Read the model definition and answer for the solid it produces. Units are mm, in the model's axes. Face numbers are marked on the shaded views. A direction names the side the tool comes from. Coordinates: 2 decimals unless noted, no trailing zeros. Loops run counter-clockwise (first coordinate to the right, second up) from the corner with the lowest first, then second, coordinate; pieces in that order, holes last. Notation, with made-up numbers: (37.25, -30.75) - (77.25, -30.75) arc R21 cw to (77.25, -9.75) - close; hole circle Ø3 at (-2, -9.5). An arc over 180 degrees is marked (long way). Use one line per item in the form item = value.
from build123d import *

# Parameters (mm, degrees)
EXTRUDE_2_DEPTH                = 5
SKETCH_4_W                     = 8.676470589
SKETCH_4_H                     = 35
SKETCH_4_W_2                   = 8.676470588
EXTRUDE_15_DEPTH               = 35
CUT_EXTRUDE_1_DEPTH            = 45
SKETCH_6_R                     = 15
CUT_EXTRUDE_2_DEPTH            = 45
FILLET_1_R                     = 5
EXTRUDE_START                  = -1
SKETCH_7_R                     = 15
SKETCH_7_R_2                   = 13
EXTRUDE_16_DEPTH               = 1
SPLIT_BODIES_1_SURFACE_1_BACK  = 86
SPLIT_BODIES_1_SURFACE_1_DEPTH = 172
SPLIT_BODIES_1_SURFACE_2_BACK  = 86
SPLIT_BODIES_1_SURFACE_2_DEPTH = 172
SKETCH_17_W                    = 3
SKETCH_17_H                    = 13
EXTRUDE_20_DEPTH               = 42
HOLE_WIZARD_1_D                = 4.3
HOLE_WIZARD_1_DEPTH            = 5
HOLE_WIZARD_1_CBORE_D          = 10
HOLE_WIZARD_1_CBORE_DEPTH      = 0.5
HOLE_WIZARD_1_TIP              = 1.291850331
EXTRUDE_21_DEPTH               = 3
SKETCH_33_R                    = 1.6
CUT_EXTRUDE_3_DEPTH            = 3
EXTRUDE_22_DEPTH               = 5
FILLET_2_R                     = 6


with BuildPart() as part:
    # 草图2 → 凸台-拉伸2 (new body)
    with BuildSketch(Plane.XY):
        Polygon((7.726423565, 24.338235294), (-14.773576435, 24.338235294), (-14.773576435, -35.661764706), (7.726423565, -35.661764706), (7.726423565, -23.161764706), (-6.097105846, -23.161764706), (-6.097105846, 11.838235294), (7.726423565, 11.838235294), align=None)
        Polygon((30.226423565, 24.338235294), (7.726423565, 24.338235294), (7.726423565, 11.838235294), (21.549952977, 11.838235294), (21.549952977, -23.161764706), (7.726423565, -23.161764706), (7.726423565, -35.661764706), (30.226423565, -35.661764706), align=None)
    extrude(amount=EXTRUDE_2_DEPTH)

    # 草图4 → 凸台-拉伸15 (add)
    with BuildSketch(Plane.XY.offset(5)):
        with Locations((-10.435341141, -5.661764706)):
            Rectangle(SKETCH_4_W, SKETCH_4_H)
        with Locations((25.888188271, -5.661764706)):
            Rectangle(SKETCH_4_W_2, SKETCH_4_H)
    extrude(amount=EXTRUDE_15_DEPTH)

    # 草图5 → 切除-拉伸1 (cut)
    with BuildSketch(Plane.ZY.offset(14.773576435)):
        with BuildLine():
            Line((40, -23.161764706), (40, -5.661764706))
            ThreePointArc((40, -5.661764706), (34.874368671, -18.036133377), (22.5, -23.161764706))
            Line((22.5, -23.161764706), (40, -23.161764706))
        make_face()
        with BuildLine():
            ThreePointArc((22.5, 11.838235294), (34.874368671, 6.712603965), (40, -5.661764706))
            Line((40, -5.661764706), (40, 11.838235294))
            Line((40, 11.838235294), (22.5, 11.838235294))
        make_face()
    extrude(amount=-CUT_EXTRUDE_1_DEPTH, mode=Mode.SUBTRACT)

    # 草图6 → 切除-拉伸2 (cut)
    with BuildSketch(Plane.ZY.offset(14.773576435)):
        with Locations((22.5, -5.661764706)):
            Circle(SKETCH_6_R)
    extrude(amount=-CUT_EXTRUDE_2_DEPTH, mode=Mode.SUBTRACT)

    # 圆角1
    fillet_1_edges = [part.edges().sort_by_distance(p)[0] for p in [
        (-6.097105846, 11.838235294, 2.5),
        (-6.097105846, -23.161764706, 2.5),
        (21.549952977, -23.161764706, 2.5),
        (21.549952977, 11.838235294, 2.5),
    ]]
    fillet(fillet_1_edges, radius=FILLET_1_R)

    # 草图7 → 凸台-拉伸16 (add)
    with BuildSketch(Plane(origin=(-6.097105846, 0, 0), x_dir=(0, 0, -1), z_dir=(1, 0, 0)).offset(EXTRUDE_START)):
        with Locations(Location((-22.5, -5.661764706, 0), (0, 0, 180))):
            Circle(SKETCH_7_R)
        with Locations((-22.5, -5.661764706)):
            Circle(SKETCH_7_R_2, mode=Mode.SUBTRACT)
    extrude(amount=EXTRUDE_16_DEPTH)


with BuildPart() as body_2:
    # Split Bodies 1: the piece behind the surface
    add(part.part)
    # Split Bodies 1 surface: a surface, the sketch's curves swept straight by 172 mm
    with BuildLine(Plane.XY.offset(5).offset(-SPLIT_BODIES_1_SURFACE_1_BACK), mode=Mode.PRIVATE) as split_bodies_1_surface_1_path:
        Line((7.726423565, 24.338235294), (7.726423565, -35.661764706))
    split_bodies_1_surface_1 = Shell.extrude(split_bodies_1_surface_1_path.wire(), (0 * SPLIT_BODIES_1_SURFACE_1_DEPTH, 0 * SPLIT_BODIES_1_SURFACE_1_DEPTH, 1 * SPLIT_BODIES_1_SURFACE_1_DEPTH))
    split(bisect_by=split_bodies_1_surface_1, keep=Keep.BOTTOM)


with BuildPart() as part_1:
    add(part.part)

    # Split Bodies 1: split by a surface, the side it looks to stays
    # Split Bodies 1 surface: a surface, the sketch's curves swept straight by 172 mm
    with BuildLine(Plane.XY.offset(5).offset(-SPLIT_BODIES_1_SURFACE_2_BACK), mode=Mode.PRIVATE) as split_bodies_1_surface_2_path:
        Line((7.726423565, 24.338235294), (7.726423565, -35.661764706))
    split_bodies_1_surface_2 = Shell.extrude(split_bodies_1_surface_2_path.wire(), (0 * SPLIT_BODIES_1_SURFACE_2_DEPTH, 0 * SPLIT_BODIES_1_SURFACE_2_DEPTH, 1 * SPLIT_BODIES_1_SURFACE_2_DEPTH))
    split(bisect_by=split_bodies_1_surface_2, keep=Keep.TOP)

    # 草图17 → 凸台-拉伸20 (add)
    with BuildSketch(Plane.XY.offset(5)):
        with Locations((28.726423565, -34.661764706)):
            Rectangle(SKETCH_17_W, SKETCH_17_H)
        with Locations((28.726423565, 25.338235294)):
            Rectangle(SKETCH_17_W, SKETCH_17_H)
    extrude(amount=EXTRUDE_20_DEPTH)

    # 打孔尺寸(%根据六角头螺)栓 全螺纹的类型1
    with Locations(Plane(origin=(18.226423565, 18.088235294, 5), x_dir=(1, 0, 0), z_dir=(0, 0, 1))):
        with Locations((0, 0), (0, -47.5)):
            CounterBoreHole(HOLE_WIZARD_1_D / 2, HOLE_WIZARD_1_CBORE_D / 2, HOLE_WIZARD_1_CBORE_DEPTH, depth=HOLE_WIZARD_1_DEPTH)
            with Locations((0, 0, -(HOLE_WIZARD_1_DEPTH + HOLE_WIZARD_1_TIP / 2))):  # 118° drill point
                Cone(0, HOLE_WIZARD_1_D / 2, HOLE_WIZARD_1_TIP, mode=Mode.SUBTRACT)

    # 草图32 → 凸台-拉伸21 (add)
    with BuildSketch(Plane(origin=(30.226423565, 0, 0), x_dir=(0, 0, -1), z_dir=(1, 0, 0))):
        with BuildLine():
            Line((-47, 31.838235294), (-47, 18.838235294))
            ThreePointArc((-47, 18.838235294), (-53.5, 25.338235294), (-47, 31.838235294))
        make_face()
        with BuildLine():
            Line((-47, -28.161764706), (-47, -41.161764706))
            ThreePointArc((-47, -41.161764706), (-53.5, -34.661764706), (-47, -28.161764706))
        make_face()
        with BuildLine():
            Line((-16.851482017, 11.838235294), (-5, 11.838235294))
            Line((-5, 11.838235294), (-5, 18.838235294))
            Line((-5, 18.838235294), (-16.851482017, 18.838235294))
            ThreePointArc((-16.851482017, 18.838235294), (-13.351482017, 15.338235294), (-16.851482017, 11.838235294))
        make_face()
        with BuildLine():
            Line((-16.851482017, -23.161764706), (-5, -23.161764706))
            Line((-5, -23.161764706), (-5, -28.161764706))
            Line((-5, -28.161764706), (-16.851482017, -28.161764706))
            ThreePointArc((-16.851482017, -28.161764706), (-14.351482017, -25.661764706), (-16.851482017, -23.161764706))
        make_face()
    extrude(amount=-EXTRUDE_21_DEPTH)

    # 草图33 → 切除-拉伸3 (cut)
    with BuildSketch(Plane(origin=(30.226423565, 0, 0), x_dir=(0, 0, -1), z_dir=(1, 0, 0))):
        with Locations((-47, 25.338235294)):
            Circle(SKETCH_33_R)
        with Locations((-47, -34.661764706)):
            Circle(SKETCH_33_R)
        with Locations((-10, 25.338235294)):
            Circle(SKETCH_33_R)
        with Locations((-10, -34.661764706)):
            Circle(SKETCH_33_R)
    extrude(amount=-CUT_EXTRUDE_3_DEPTH, mode=Mode.SUBTRACT)

    # 草图34 → 凸台-拉伸22 (add)
    with BuildSketch(Plane.XY.offset(5)):
        Polygon((18.226423565, 24.338235294), (30.226423565, 24.338235294), (30.226423565, 35.338235294), align=None)
        Polygon((18.226423565, -35.661764706), (30.226423565, -35.661764706), (30.226423565, -43.661764706), align=None)
    extrude(amount=-EXTRUDE_22_DEPTH)

    # 圆角2
    fillet_2_edges = [part_1.edges().sort_by_distance(p)[0] for p in [
        (18.226423565, 24.338235294, 2.5),
        (18.226423565, -35.661764706, 2.5),
    ]]
    fillet(fillet_2_edges, radius=FILLET_2_R)


solid = part_1.part
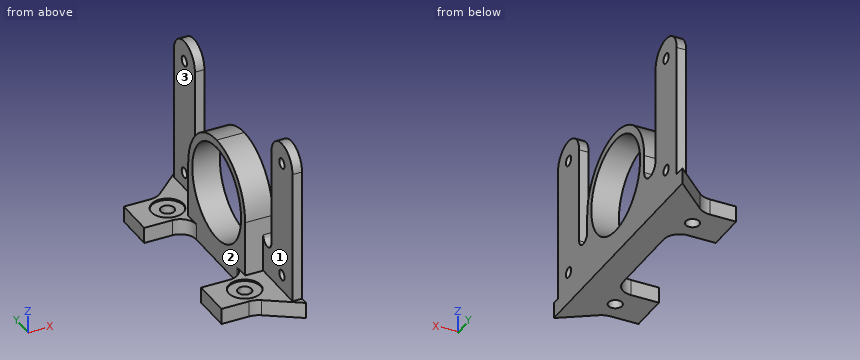
Item 1: The part is cut by section B-B on y = 4. Give the vertices of the cut face in (x, z).
Results below:
outline = (21.55, 0) - (30.23, 0) - (30.23, 11.03) - (21.55, 11.03) - close; (21.55, 33.97) - (30.23, 33.97) - (30.23, 37.09) - (21.55, 37.09) - close
Item 2: Find the intervals of material crossed by L1, parallel to Y at x = 28.05, z = 47; L2, parallel to Y at x = 28.6, z = 10; L3, parallel to Y at x = 23.75, z = 23, in increasing order.
Results below:
L1 = -41.16 to -36.26, -33.06 to -28.16, 18.84 to 23.74, 26.94 to 31.84
L2 = -41.16 to -36.26, -33.06 to -13.95, 2.63 to 23.74, 26.94 to 31.84
L3 = -23.15 to -20.65, 9.33 to 11.83
Item 3: The part is cut by section C-C on z = 19. Give the vertices of the cut face in (x, y), plus the area to 3 significant figures.
Results below:
outline = (21.55, -23.16) - (30.23, -23.16) - (30.23, -20.25) - (21.55, -20.25) - close; (21.55, 8.92) - (30.23, 8.92) - (30.23, 11.84) - (21.55, 11.84) - close; (27.23, -41.16) - (30.23, -41.16) - (30.23, -28.16) - (27.23, -28.16) - close; (27.23, 18.84) - (30.23, 18.84) - (30.23, 31.84) - (27.23, 31.84) - close
area = 129 mm²
Item 4: The part is cut by section D-D on y = 21.5. Give the vertices of the cut face in (x, z), plus the area to 3 significant figures.
Results below:
outline = (7.73, 0) - (30.23, 0) - (30.23, 52.25) - (27.23, 52.25) - (27.23, 5) - (21.88, 5) - (21.88, 4.5) - (14.57, 4.5) - (14.57, 5) - (7.73, 5) - close
area = 251 mm²
Item 5: Each of these flat-tipped pins is pushed along its axis until it touches: P1, Ø4, axis at x = 27, z = 24, coming from the +Y side; P2, Ø5, axis at x = 23, y = 26, coming from the +Z side; P3, Ø10, axis at y = 18.5, z = 40, coming from the -X side. Where does it stop, or does it pass through?
Results below:
P1 = 31.84
P2 = 5
P3 = 27.23
Item 6: The part is cut by section A-A on x = 12. Give the vertices of the cut face in (y, z).
Results below:
outline = (-35.66, 0) - (-23.16, 0) - (-23.16, 5) - (-35.66, 5) - close; (11.84, 0) - (24.34, 0) - (24.34, 5) - (11.84, 5) - close
Item 7: Which of the six approach directions +Z, -Z, +X, -X, +Y, -Y give full straight-line access (tool end or side, diameter ignored) to the marked faces 1, 2 and 3?
Results below:
face_1 = +Z, -X, -Y
face_2 = +Z, -X
face_3 = +Z, -X, +Y
